Drawing for the job (mm, zero at the part's lowest x, y, z). A direction names the side the tool comes from. Give positions to 0.01 mm unless a question says otherwise; leave off trailing zeros. Order: outer loops, then holes, each group sorted by start corner. A loop starts at its lowest first (then second) coordinate and runs counter-clockwise, first axis right, second up. Notation, with made-up numbers: (-28, 41) -> (-24, 41) arc R17 ccw to (-24, 67) -> close; hole circle Ø1 at (1.5, 19.25). An arc over 180 degrees is marked (long way). Use one line per item in the form item = value. Start each with the question number.
1) Cut at D-D, the plane y = 13. Give the cut face in (x, z), and give its area (3 significant figures).
2) Cut at A-A, the plane z = 2.5. Give the cut face in (x, y), and give its area (3 significant figures).
3) Drop flat-ended pins along their axis: P1, Ø2, axis at x = 4, z = 17.5, coming from the +Y side; P2, Ø1.5, axis at x = 5, z = 24, coming from the -Y side; P3, Ø1.5, axis at y = 11.5, z = 22, coming from the +X side (1 decimal). Give the stop position or say it passes through.
4) Cut at C-C, the plane x = 5. Give the cut face in (y, z), and give its area (3 significant figures).
5) Probe line 1 (Z direction, x = 5.25, y = 2.5); line 2 (Z direction, x = 11.5, y = 9); line 3 (X direction, y = 2.75, z = 20) (1 decimal). List the from-to ranges inside material, lowest first.
6) Cut at B-B, the plane y = 4.25. Give the cut face in (x, z).
7) Tool access for the marked faces 1 and 2: list every direction of +Z, -Z, +X, -X, +Y, -Y with a clear straight run to the whole face (end or side of a thin tool).
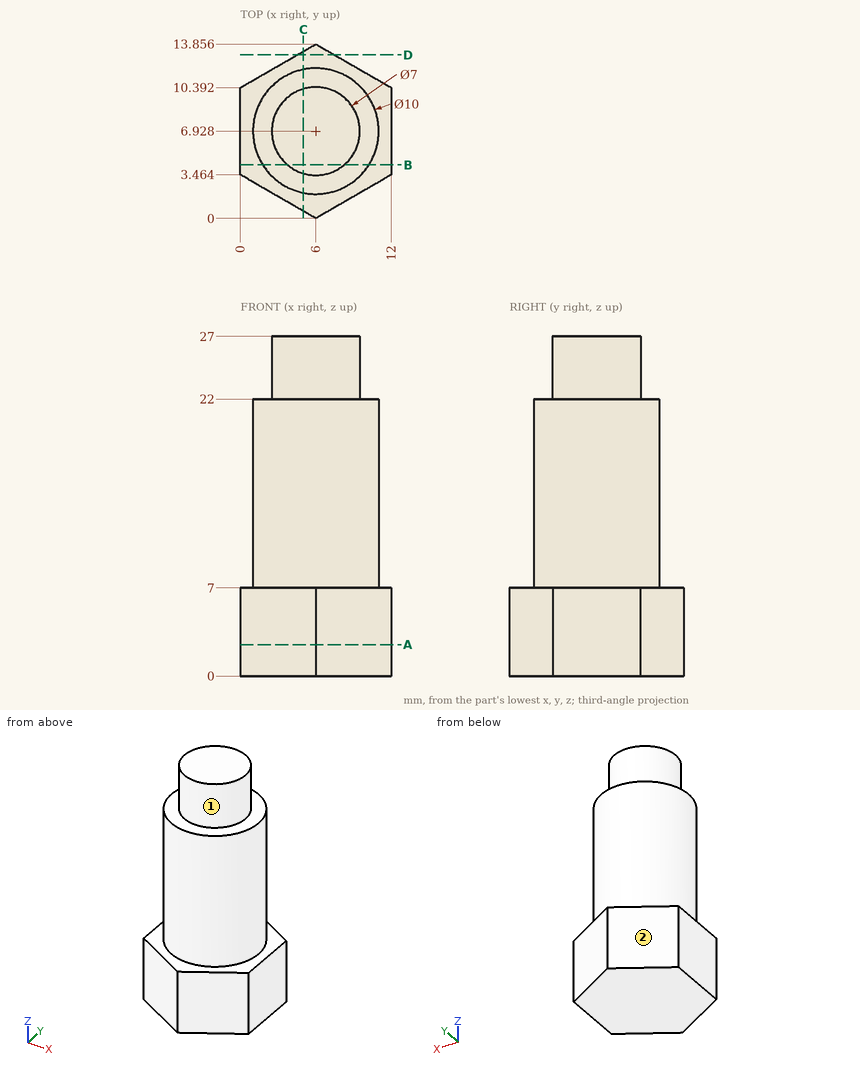
Result:
q1.outline = (4.52, 0) -> (7.48, 0) -> (7.48, 7) -> (4.52, 7) -> close
q1.area = 20.8 mm²
q2.outline = (0, 3.46) -> (6, 0) -> (12, 3.46) -> (12, 10.39) -> (6, 13.86) -> (0, 10.39) -> close
q2.area = 125 mm²
q3.P1 = 11.83
q3.P2 = 3.44
q3.P3 = 9.2
q4.outline = (0.58, 0) -> (13.28, 0) -> (13.28, 7) -> (11.83, 7) -> (11.83, 22) -> (10.28, 22) -> (10.28, 27) -> (3.57, 27) -> (3.57, 22) -> (2.03, 22) -> (2.03, 7) -> (0.58, 7) -> close
q4.area = 269 mm²
q5.line_1 = 0 to 22
q5.line_2 = 0 to 7
q5.line_3 = 3.3 to 8.7
q6.outline = (0, 0) -> (12, 0) -> (12, 7) -> (10.22, 7) -> (10.22, 22) -> (8.25, 22) -> (8.25, 27) -> (3.75, 27) -> (3.75, 22) -> (1.78, 22) -> (1.78, 7) -> (0, 7) -> close
q7.face_1 = +Z
q7.face_2 = +Z, -Z, -X, +Y
